Geometry: final body of the model. Coordinates: model frame, mm. Face numbers are marked on the shaded views. Round coordinates to 2 decimals unless told otherwise and drop trailing zeros. Write each loop counter-clockwise with the first axis right and the second up, starting at its lowest first coordinate (ties: lowest second). Pieces come first, ordered by that corner, then holes. Notation, with made-up numbers: (33.25, 80) - (86.25, 80) arc R19 ccw to (86.25, 117) - close; hole circle Ø6 at (-37, 65). An arc over 180 degrees is marked (long way). Use a Markdown table: item, result. Add a question column.
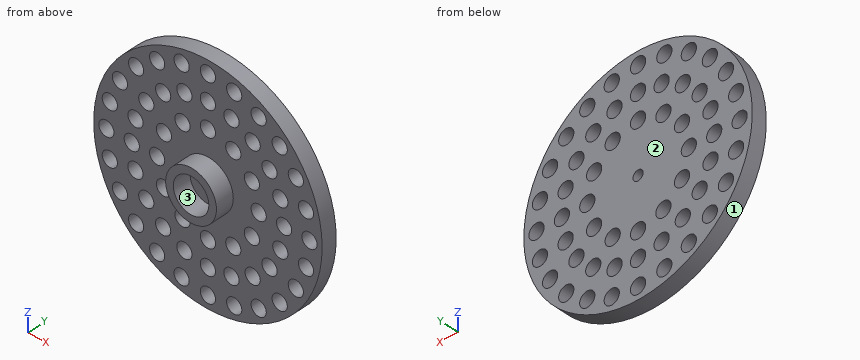
```python
from build123d import *

# Parameters (mm, degrees)
ESBO_O1_R                = 5
ESBO_O1_R_2              = 3.5
RESSALTO_EXTRUS_O1_DEPTH = 3.6
ESBO_O4_R                = 22.5
RESSALTO_EXTRUS_O2_DEPTH = 3
ESBO_O5_R                = 1
ESBO_O5_R_2              = 1.5
CORTE_EXTRUS_O2_DEPTH    = 7.6


with BuildPart() as part:
    # Esboço1 → Ressalto-extrusão1 (new body)
    with BuildSketch(Plane(origin=(0, 0, 0), x_dir=(1, 0, 0), z_dir=(0, 1, 0))):
        Circle(ESBO_O1_R)
        Circle(ESBO_O1_R_2, mode=Mode.SUBTRACT)
    extrude(amount=RESSALTO_EXTRUS_O1_DEPTH)

    # Esboço4 → Ressalto-extrusão2 (add)
    with BuildSketch(Plane(origin=(0, 3.6, 0), x_dir=(1, 0, 0), z_dir=(0, 1, 0))):
        Circle(ESBO_O4_R)
    extrude(amount=RESSALTO_EXTRUS_O2_DEPTH)

    # Esboço5 → Corte-extrusão2 (cut, through all)
    with BuildSketch(Plane(origin=(0, 6.6, 0), x_dir=(1, 0, 0), z_dir=(0, 1, 0))):
        Circle(ESBO_O5_R)
        with Locations((0, 20)):
            Circle(ESBO_O5_R_2)
        with Locations((0, 15)):
            Circle(ESBO_O5_R_2)
        with Locations((0, 10)):
            Circle(ESBO_O5_R_2)
        with Locations((5, 8.660254038)):
            Circle(ESBO_O5_R_2)
        with Locations((8.660254038, 5)):
            Circle(ESBO_O5_R_2)
        with Locations((10, 0)):
            Circle(ESBO_O5_R_2)
        with Locations((8.660254038, -5)):
            Circle(ESBO_O5_R_2)
        with Locations((5, -8.660254038)):
            Circle(ESBO_O5_R_2)
        with Locations((0, -10)):
            Circle(ESBO_O5_R_2)
        with Locations((-5, -8.660254038)):
            Circle(ESBO_O5_R_2)
        with Locations((-8.660254038, -5)):
            Circle(ESBO_O5_R_2)
        with Locations((-10, 0)):
            Circle(ESBO_O5_R_2)
        with Locations((-8.660254038, 5)):
            Circle(ESBO_O5_R_2)
        with Locations((-5, 8.660254038)):
            Circle(ESBO_O5_R_2)
        with Locations((4.635254916, 14.265847744)):
            Circle(ESBO_O5_R_2)
        with Locations((8.816778784, 12.135254916)):
            Circle(ESBO_O5_R_2)
        with Locations((12.135254916, 8.816778784)):
            Circle(ESBO_O5_R_2)
        with Locations((14.265847744, 4.635254916)):
            Circle(ESBO_O5_R_2)
        with Locations((15, 0)):
            Circle(ESBO_O5_R_2)
        with Locations((14.265847744, -4.635254916)):
            Circle(ESBO_O5_R_2)
        with Locations((12.135254916, -8.816778784)):
            Circle(ESBO_O5_R_2)
        with Locations((8.816778784, -12.135254916)):
            Circle(ESBO_O5_R_2)
        with Locations((4.635254916, -14.265847744)):
            Circle(ESBO_O5_R_2)
        with Locations((0, -15)):
            Circle(ESBO_O5_R_2)
        with Locations((-4.635254916, -14.265847744)):
            Circle(ESBO_O5_R_2)
        with Locations((-8.816778784, -12.135254916)):
            Circle(ESBO_O5_R_2)
        with Locations((-12.135254916, -8.816778784)):
            Circle(ESBO_O5_R_2)
        with Locations((-14.265847744, -4.635254916)):
            Circle(ESBO_O5_R_2)
        with Locations((-15, 0)):
            Circle(ESBO_O5_R_2)
        with Locations((-14.265847744, 4.635254916)):
            Circle(ESBO_O5_R_2)
        with Locations((-12.135254916, 8.816778784)):
            Circle(ESBO_O5_R_2)
        with Locations((-8.816778784, 12.135254916)):
            Circle(ESBO_O5_R_2)
        with Locations((-4.635254916, 14.265847744)):
            Circle(ESBO_O5_R_2)
        with Locations((5.176380902, 19.318516526)):
            Circle(ESBO_O5_R_2)
        with Locations((10, 17.320508076)):
            Circle(ESBO_O5_R_2)
        with Locations((14.142135624, 14.142135624)):
            Circle(ESBO_O5_R_2)
        with Locations((17.320508076, 10)):
            Circle(ESBO_O5_R_2)
        with Locations((19.318516526, 5.176380902)):
            Circle(ESBO_O5_R_2)
        with Locations((20, 0)):
            Circle(ESBO_O5_R_2)
        with Locations((19.318516526, -5.176380902)):
            Circle(ESBO_O5_R_2)
        with Locations((17.320508076, -10)):
            Circle(ESBO_O5_R_2)
        with Locations((14.142135624, -14.142135624)):
            Circle(ESBO_O5_R_2)
        with Locations((10, -17.320508076)):
            Circle(ESBO_O5_R_2)
        with Locations((5.176380902, -19.318516526)):
            Circle(ESBO_O5_R_2)
        with Locations((0, -20)):
            Circle(ESBO_O5_R_2)
        with Locations((-5.176380902, -19.318516526)):
            Circle(ESBO_O5_R_2)
        with Locations((-10, -17.320508076)):
            Circle(ESBO_O5_R_2)
        with Locations((-14.142135624, -14.142135624)):
            Circle(ESBO_O5_R_2)
        with Locations((-17.320508076, -10)):
            Circle(ESBO_O5_R_2)
        with Locations((-19.318516526, -5.176380902)):
            Circle(ESBO_O5_R_2)
        with Locations((-20, 0)):
            Circle(ESBO_O5_R_2)
        with Locations((-19.318516526, 5.176380902)):
            Circle(ESBO_O5_R_2)
        with Locations((-17.320508076, 10)):
            Circle(ESBO_O5_R_2)
        with Locations((-14.142135624, 14.142135624)):
            Circle(ESBO_O5_R_2)
        with Locations((-10, 17.320508076)):
            Circle(ESBO_O5_R_2)
        with Locations((-5.176380902, 19.318516526)):
            Circle(ESBO_O5_R_2)
    extrude(amount=-CORTE_EXTRUS_O2_DEPTH, mode=Mode.SUBTRACT)


solid = part.part
```
1) Section A-A, the plane x = -15. Return the cut outline in (y, z).
2) Section B-B, the plane z = 20. Return the cut outline in (x, y), then the cut area to 3 significant figures.
3) Section D-D, the plane z = 15. Return the cut outline in (x, y), then the cut area to 3 significant figures.
4) Section C-C, the plane x = 20. Return the cut outline in (y, z), then the cut area to 3 significant figures.
5) Material intervals for L1, parallel to X at y = 6.25, z = -11; L2, parallel to X at y = 5.55, z = 15; L3, parallel to Z at x = -20, y = 5.5, sorted ascending. Write a range as from..to.
6) Pin query (flat end, axial travel): P1, Ø5, axis at x = -17.32, z = -10, coming from the -Y side. Return the tip coordinate at first contact, or that it passes through.
7) Draft query along Z for the marked faces 1, 2 and 3. Return one class per face: released by +Z, released by -Z, zero draft, split by the parting line, or undercut.
Output values:
| question | item | result |
|---|---|---|
| 1 | outline | (3.6, -16.77) - (6.6, -16.77) - (6.6, -15.37) - (3.6, -15.37) - close; (3.6, -12.91) - (6.6, -12.91) - (6.6, -5.94) - (3.6, -5.94) - close; (3.6, -3.33) - (6.6, -3.33) - (6.6, -1.5) - (3.6, -1.5) - close; (3.6, 1.5) - (6.6, 1.5) - (6.6, 3.33) - (3.6, 3.33) - close; (3.6, 5.94) - (6.6, 5.94) - (6.6, 12.91) - (3.6, 12.91) - close; (3.6, 15.37) - (6.6, 15.37) - (6.6, 16.77) - (3.6, 16.77) - close |
| 2 | outline | (-10.31, 3.6) - (-6.51, 3.6) - (-6.51, 6.6) - (-10.31, 6.6) - close; (-3.84, 3.6) - (-1.5, 3.6) - (-1.5, 6.6) - (-3.84, 6.6) - close; (1.5, 3.6) - (3.84, 3.6) - (3.84, 6.6) - (1.5, 6.6) - close; (6.51, 3.6) - (10.31, 3.6) - (10.31, 6.6) - (6.51, 6.6) - close |
| 2 | area | 36.8 mm^2 |
| 3 | outline | (-16.77, 3.6) - (-15.37, 3.6) - (-15.37, 6.6) - (-16.77, 6.6) - close; (-12.91, 3.6) - (-5.94, 3.6) - (-5.94, 6.6) - (-12.91, 6.6) - close; (-3.33, 3.6) - (-1.5, 3.6) - (-1.5, 6.6) - (-3.33, 6.6) - close; (1.5, 3.6) - (3.33, 3.6) - (3.33, 6.6) - (1.5, 6.6) - close; (5.94, 3.6) - (12.91, 3.6) - (12.91, 6.6) - (5.94, 6.6) - close; (15.37, 3.6) - (16.77, 3.6) - (16.77, 6.6) - (15.37, 6.6) - close |
| 3 | area | 61.2 mm^2 |
| 4 | outline | (3.6, -10.31) - (6.6, -10.31) - (6.6, -6.51) - (3.6, -6.51) - close; (3.6, -3.84) - (6.6, -3.84) - (6.6, -1.5) - (3.6, -1.5) - close; (3.6, 1.5) - (6.6, 1.5) - (6.6, 3.84) - (3.6, 3.84) - close; (3.6, 6.51) - (6.6, 6.51) - (6.6, 10.31) - (3.6, 10.31) - close |
| 4 | area | 36.8 mm^2 |
| 5 | L1 | x = -19.63..-18.44, -16.2..-9.8, -7.84..-1.12, 1.12..7.84, 9.8..16.2, 18.44..19.63 |
| 5 | L2 | x = -16.77..-15.37, -12.91..-5.94, -3.33..-1.5, 1.5..3.33, 5.94..12.91, 15.37..16.77 |
| 5 | L3 | z = -10.31..-6.51, -3.84..-1.5, 1.5..3.84, 6.51..10.31 |
| 6 | P1 | stops at y = 3.6 |
| 7 | face 1 | split by the parting line |
| 7 | face 2 | zero draft |
| 7 | face 3 | undercut |
